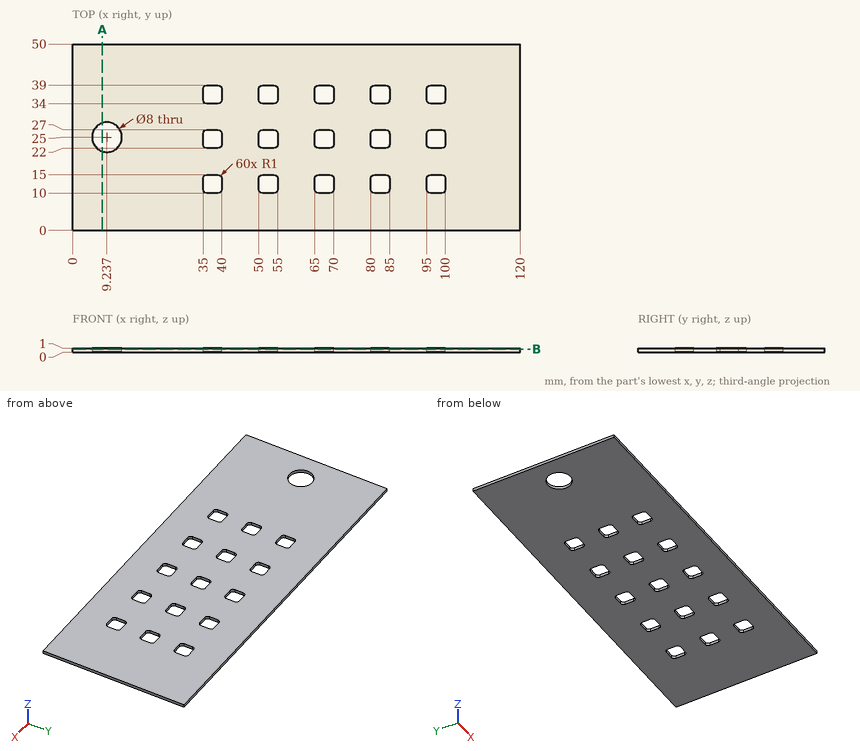
Design review of the part shown in the three views and the two pictorial views. Dimensions are in mm from the part's minimum x, y and z. Round coordinates to 2 decimals unless told otherwise and drop trailing zeros. Write each loop counter-clockwise with the first axis right and the second up, starting at its lowest first coordinate (ties: lowest second). Pieces come first, ordered by that corner, then holes. Notation, with made-up numbers: (-31.75, -34.75) - (-15.75, -34.75) arc R6 cw to (-15.75, -23.75) - close; hole circle Ø10 at (2, 22.25). An arc over 180 degrees is marked (long way). Write item = value, one per line. Start each with the question number.
1. Wall thickness on L1, parallel to Y at x = 96, z = 0.25; L2, parallel to X at y = 35.5, z = 0.3; L3, parallel to X at y = 28, z = 0.75 (1 decimal): over which ranges is each line inside the solid? List them lowest first.
2. Consider section B-B on z = 0.8. Give the number of separate pieces and of enclosed holes in the cut face, plus the area to 3 significant figures.
3. For pin 1 Ø1 at (x, y) = (73.5, 21) entering from -Z, flat-tipped, find the tip position at first contact; note if it passes through.
4. Consider section A-A on x = 8. State the section outline as (y, z) points.
Evaluation:
q1.L1 = 0 to 10, 15 to 22, 27 to 34, 39 to 50
q1.L2 = 0 to 35, 40 to 50, 55 to 65, 70 to 80, 85 to 95, 100 to 120
q1.L3 = 0 to 6.6, 11.9 to 120
q2.separate_pieces = 1
q2.enclosed_holes = 16
q2.area = 5,590 mm2
q3.pin_1 = 0
q4.outline = (0, 0) - (21.2, 0) - (21.2, 1) - (0, 1) - close; (28.8, 0) - (50, 0) - (50, 1) - (28.8, 1) - close
